The figure shows three views and two pictorial views of one solid part (mm, origin at its lowest corner). Answer the questions. Coordinates: 2 decimals unless noted, no trailing zeros. Order: outer loops, then holes, each group sorted by start corner. A loop starts at its lowest first (then second) coordinate and runs counter-clockwise, first axis right, second up. Notation, with made-up numbers: (-20.75, 44.25) -> (16.25, 44.25) arc R28 ccw to (16.25, 65.25) -> close; hole circle Ø4 at (17, 21). An arc over 180 degrees is marked (long way). Write item = value, one per line. Start each with the question number.
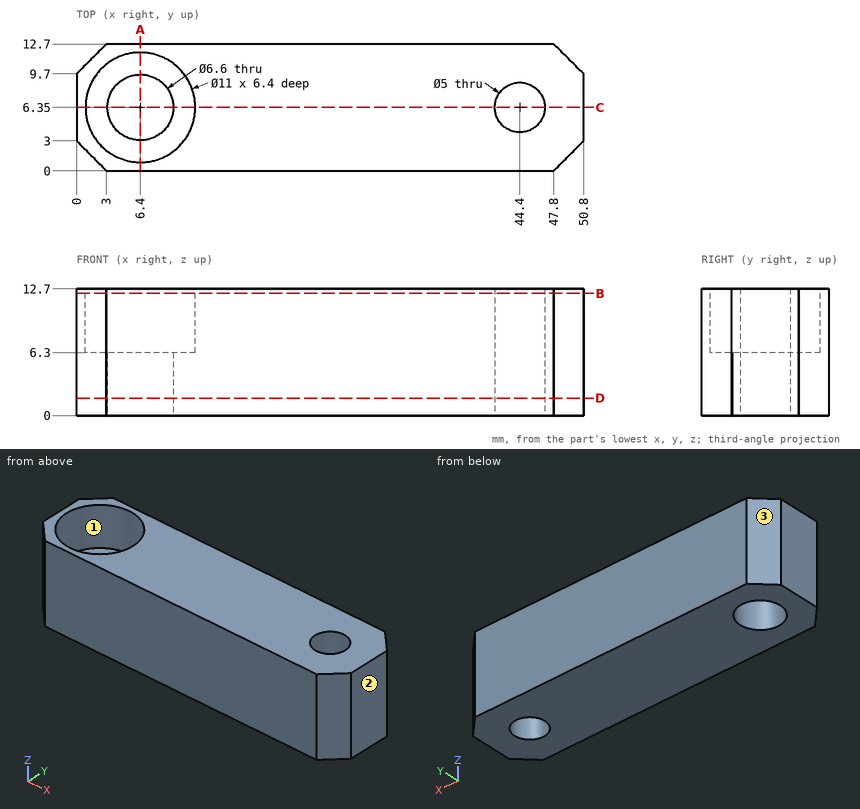
Item 1: Section B-B, the plane z = 12.25 is taken. Give the vertices of the cut face in (x, y).
Item 2: Consider probe 1 along Y at (x, z) = (6.4, 7.75); probe 2 along X at (y, z) = (7.25, 8.25); probe 3 along Y at (x, z) = (6.4, 1.5). Determine where each line is inside the solid, lowest interval first.
Item 3: Section C-C, the plane y = 6.35 is taken. Give the vertices of the cut face in (x, z).
Item 4: Section D-D, the plane z = 1.75 is taken. Give the vertices of the cut face in (x, y), then the cut area to 3 significant figures.
Item 5: For a pull along X with two mould halves and no side action, classify the marked faces 1, 2 and 3 as pulls with the +X half, pulls with the -X half, needs draft (parallel to the pull), parting line crosses it, or undercut.
Item 6: Section A-A, the plane x = 6.4 is taken. Give the vertices of the cut face in (y, z), then the cut area to 3 significant figures.
A:
q1.outline = (0, 3) -> (3, 0) -> (47.8, 0) -> (50.8, 3) -> (50.8, 9.7) -> (47.8, 12.7) -> (3, 12.7) -> (0, 9.7) -> close; hole circle Ø11 at (6.4, 6.35); hole circle Ø5 at (44.4, 6.35)
q2.probe_1 = 0 to 0.85, 11.85 to 12.7
q2.probe_2 = 0 to 0.97, 11.83 to 42.07, 46.73 to 50.8
q2.probe_3 = 0 to 3.05, 9.65 to 12.7
q3.outline = (0, 0) -> (3.1, 0) -> (3.1, 6.3) -> (0.9, 6.3) -> (0.9, 12.7) -> (0, 12.7) -> close; (9.7, 0) -> (41.9, 0) -> (41.9, 12.7) -> (11.9, 12.7) -> (11.9, 6.3) -> (9.7, 6.3) -> close; (46.9, 0) -> (50.8, 0) -> (50.8, 12.7) -> (46.9, 12.7) -> close
q4.outline = (0, 3) -> (3, 0) -> (47.8, 0) -> (50.8, 3) -> (50.8, 9.7) -> (47.8, 12.7) -> (3, 12.7) -> (0, 9.7) -> close; hole circle Ø6.6 at (6.4, 6.35); hole circle Ø5 at (44.4, 6.35)
q4.area = 573 mm^2
q5.face_1 = undercut
q5.face_2 = pulls with the +X half
q5.face_3 = pulls with the -X half
q6.outline = (0, 0) -> (3.05, 0) -> (3.05, 6.3) -> (0.85, 6.3) -> (0.85, 12.7) -> (0, 12.7) -> close; (9.65, 0) -> (12.7, 0) -> (12.7, 12.7) -> (11.85, 12.7) -> (11.85, 6.3) -> (9.65, 6.3) -> close
q6.area = 49.3 mm^2
